For this review, use the dimensioned drawing (mm, ordinates from the lowest corner) and the shaded views. Coordinates: 2 decimals unless noted, no trailing zeros. Loops run counter-clockwise (first coordinate to the right, second up) from the corner with the lowest first, then second, coordinate; pieces in that order, holes last. Notation, with made-up numbers: (56.25, 66) - (71.25, 66) arc R23 cw to (71.25, 82) - close; hole circle Ø8 at (52, -16). An arc over 180 degrees is marked (long way). One line per item, written item: value. Start each with the question number.
1. We need section C-C, the plane z = 29. Give the boundary of the cut face in (x, y), then the cut area to 3 significant figures.
2. We need section B-B, the plane y = 186.5. Give the boundary of the cut face in (x, z).
3. We need section A-A, the plane x = 1.8. Give the boundary of the cut face in (y, z).
4. Insertion check: P1, Ø1.5, axis at x = 2, y = 64.5, coming from the +Z side; P2, Ø1.5, axis at x = 2, z = 35, coming from the -Y side; P3, Ø1, axis at x = 1.5, y = 258.5, coming from the -Z side. Each pin has a flat end and moves straight along its axis. Give the tip position at first contact, or say it passes through.
5. To check wall thickness, follow line 1 (Z direction, x = 1.55, y = 189.5); line 2 (Y direction, x = 1.9, z = 34.5); line 3 (Z direction, x = 1.25, y = 276.5). State the ranges of each line that lie inside material, in increasing order.
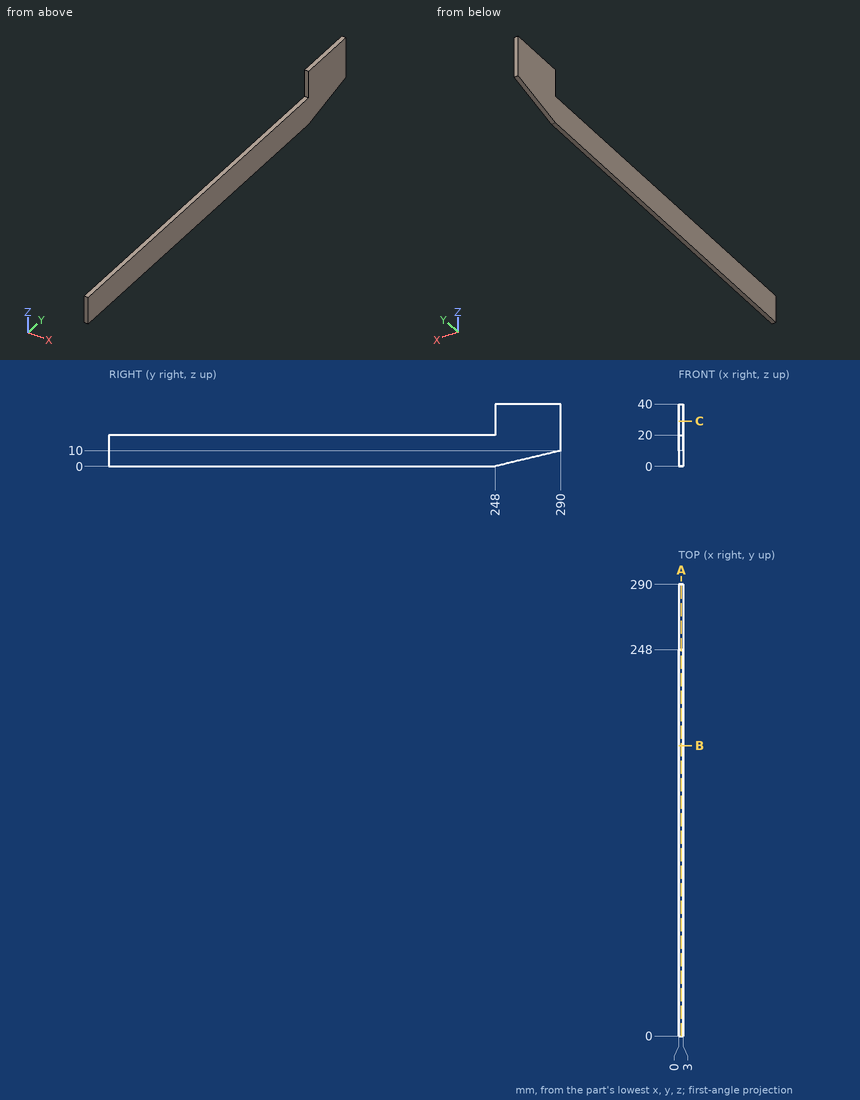
Findings below:
1. outline: (0, 248) - (3, 248) - (3, 290) - (0, 290) - close
1. area: 126 mm2
2. outline: (0, 0) - (3, 0) - (3, 20) - (0, 20) - close
3. outline: (0, 0) - (248, 0) - (290, 10) - (290, 40) - (248, 40) - (248, 20) - (0, 20) - close
4. P1: z = 20
4. P2: y = 248
4. P3: z = 2.38
5. line 1: 0 to 20
5. line 2: 248 to 290
5. line 3: 6.79 to 40
